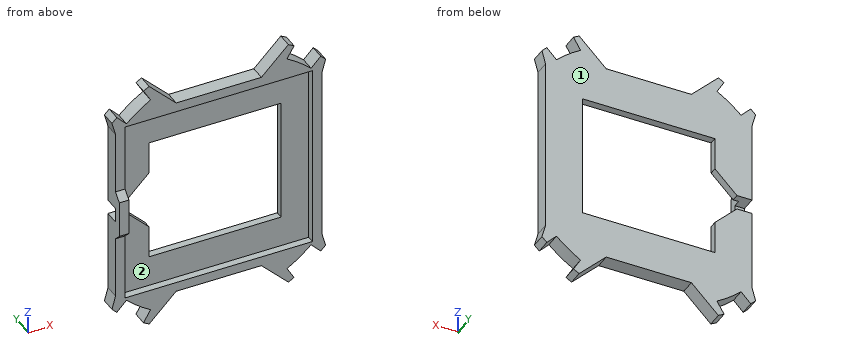
```python
from build123d import *

# Parameters (mm, degrees)
BOSS_EXTRUDE3_DEPTH      = 1
BOSS_EXTRUDE3_DEPTH_BACK = 1
SKETCH3_W                = 18
SKETCH3_H                = 17
CUT_EXTRUDE1_DEPTH       = 23.944525539
SKETCH3_4_W              = 25.5
SKETCH3_4_H              = 25.5
SKETCH3_4_W_2            = 18
SKETCH3_4_H_2            = 17
CUT_EXTRUDE3_DEPTH       = 23.944525539
CUT_EXTRUDE4_DEPTH       = 23.944525539
CUT_EXTRUDE4_DEPTH_BACK  = 23.944525539
SKETCH4_W                = 16
SKETCH4_H                = 2
CHAMFER1_SIZE            = 3
SKETCH6_W                = 5
SKETCH6_H                = 1
BOSS_EXTRUDE5_DEPTH      = 1.3
CHAMFER2_SIZE            = 1


with BuildPart() as part:
    # Sketch2 → Boss-Extrude3 (new, two sides: drawn at the far end of the back side and taken through both)
    with BuildSketch(Plane(origin=(0, -16.832566415, 0), x_dir=(1, 0, 0), z_dir=(0, 1, 0)).offset(-BOSS_EXTRUDE3_DEPTH_BACK)):
        with BuildLine():
            Line((14.05, -12.05), (14.05, 12.05))
            Line((14.05, 12.05), (14.538378439, 13.872653149))
            ThreePointArc((14.538378439, 13.872653149), (14.210517369, 14.208312678), (13.874908715, 14.536225824))
            Line((13.874908715, 14.536225824), (12.56303347, 13.16182292))
            ThreePointArc((12.56303347, 13.16182292), (10.992315824, 14.499392587), (9.280277793, 15.650553876))
            Line((9.280277793, 15.650553876), (10.249356378, 17.284838642))
            ThreePointArc((10.249356378, 17.284838642), (9.863353095, 17.507975862), (9.47249431, 17.72249431))
            Line((9.47249431, 17.72249431), (5.8, 14.05))
            Line((5.8, 14.05), (-5.8, 14.05))
            Line((-5.8, 14.05), (-9.47249431, 17.72249431))
            ThreePointArc((-9.47249431, 17.72249431), (-9.863353095, 17.507975862), (-10.249356378, 17.284838642))
            Line((-10.249356378, 17.284838642), (-9.280277793, 15.650553876))
            ThreePointArc((-9.280277793, 15.650553876), (-10.992315824, 14.499392587), (-12.56303347, 13.16182292))
            Line((-12.56303347, 13.16182292), (-13.874908715, 14.536225824))
            ThreePointArc((-13.874908715, 14.536225824), (-14.210517369, 14.208312678), (-14.538378439, 13.872653149))
            Line((-14.538378439, 13.872653149), (-14.05, 12.05))
            Line((-14.05, 12.05), (-14.05, -12.05))
            Line((-14.05, -12.05), (-14.538378439, -13.872653149))
            ThreePointArc((-14.538378439, -13.872653149), (-14.210517369, -14.208312678), (-13.874908715, -14.536225824))
            Line((-13.874908715, -14.536225824), (-12.56303347, -13.16182292))
            ThreePointArc((-12.56303347, -13.16182292), (-10.992315824, -14.499392587), (-9.280277793, -15.650553876))
            Line((-9.280277793, -15.650553876), (-10.249356378, -17.284838642))
            ThreePointArc((-10.249356378, -17.284838642), (-9.863353095, -17.507975862), (-9.47249431, -17.72249431))
            Line((-9.47249431, -17.72249431), (-5.8, -14.05))
            Line((-5.8, -14.05), (5.8, -14.05))
            Line((5.8, -14.05), (9.47249431, -17.72249431))
            ThreePointArc((9.47249431, -17.72249431), (9.863353095, -17.507975862), (10.249356378, -17.284838642))
            Line((10.249356378, -17.284838642), (9.280277793, -15.650553876))
            ThreePointArc((9.280277793, -15.650553876), (10.992315824, -14.499392587), (12.56303347, -13.16182292))
            Line((12.56303347, -13.16182292), (13.874908715, -14.536225824))
            ThreePointArc((13.874908715, -14.536225824), (14.210517369, -14.208312678), (14.538378439, -13.872653149))
            Line((14.538378439, -13.872653149), (14.05, -12.05))
        make_face()
    extrude(amount=BOSS_EXTRUDE3_DEPTH + BOSS_EXTRUDE3_DEPTH_BACK)

    # Sketch3 → Cut-Extrude1 (cut, through all)
    with BuildSketch(Plane(origin=(0, -16.832566415, 0), x_dir=(1, 0, 0), z_dir=(0, 1, 0))):
        Rectangle(SKETCH3_W, SKETCH3_H)
    extrude(amount=CUT_EXTRUDE1_DEPTH, mode=Mode.SUBTRACT)

    # Sketch3<4> → Cut-Extrude3 (cut, through all)
    # profile 1 of 2: a face of its own
    with BuildSketch(Plane(origin=(0, -16.832566415, 0), x_dir=(1, 0, 0), z_dir=(0, 1, 0))):
        Rectangle(SKETCH3_4_W, SKETCH3_4_H)
        Rectangle(SKETCH3_4_W_2, SKETCH3_4_H_2, mode=Mode.SUBTRACT)
    # profile 2 of 2: a face of its own
    with BuildSketch(Plane(origin=(0, -16.832566415, 0), x_dir=(1, 0, 0), z_dir=(0, 1, 0))):
        Rectangle(SKETCH3_4_W_2, SKETCH3_4_H_2)
    extrude(amount=-CUT_EXTRUDE3_DEPTH, mode=Mode.SUBTRACT)

    # Sketch4 → Cut-Extrude4 (cut, two sides: drawn at the far end of the back side and taken through both)
    with BuildSketch(Plane(origin=(0, -16.832566415, 0), x_dir=(1, 0, 0), z_dir=(0, 1, 0)).offset(-CUT_EXTRUDE4_DEPTH_BACK)):
        with Locations((-13.844488576, 0)):
            Rectangle(SKETCH4_W, SKETCH4_H)
    extrude(amount=CUT_EXTRUDE4_DEPTH + CUT_EXTRUDE4_DEPTH_BACK, mode=Mode.SUBTRACT)

    # Chamfer1
    chamfer1_edges = [part.edges().sort_by_distance(p)[0] for p in [
        (-9, -16.332566415, -1),
        (-9, -16.332566415, 1),
    ]]
    chamfer(chamfer1_edges, length=CHAMFER1_SIZE)

    # Sketch6 → Boss-Extrude5 (add)
    with BuildSketch(Plane.ZY.offset(14.05)):
        with Locations((0, -18.332566415)):
            Rectangle(SKETCH6_W, SKETCH6_H)
    extrude(amount=-BOSS_EXTRUDE5_DEPTH)

    # Chamfer2
    chamfer2_edges = [part.edges().sort_by_distance(p)[0] for p in [
        (-13.4, -17.832566415, 2.5),
        (-13.4, -17.832566415, -2.5),
    ]]
    chamfer(chamfer2_edges, length=CHAMFER2_SIZE - 0.0001)  # a hair under: the kernel refuses the full size


solid = part.part
```
Here's how the part is built. I have some questions about the finished solid (model axes, mm). Face numbers are marked on the shaded views. Coordinates: 2 decimals unless noted, no trailing zeros. Order: outer loops, then holes, each group sorted by start corner. A loop starts at its lowest first (then second) coordinate and runs counter-clockwise, first axis right, second up.
Item 1: If we section it at C-C, the plane z = -11: List the corners of the cut face in (x, y) for me, then the cut area to 3 significant figures.
Response values:
outline: (-14.05, -17.83) - (-12.75, -17.83) - (-12.75, -16.83) - (12.75, -16.83) - (12.75, -17.83) - (14.05, -17.83) - (14.05, -15.83) - (-14.05, -15.83) - close
area: 30.7 mm2
Item 2: I need wall thicknesses on probe 1 along X at (y, z) = (-17.2, 5); probe 2 along Y at (x, z) = (-10, 10.5). Which ranges of each line are inside material? Lowest first, please.
Response values:
probe 1: x = -14.05 to -12.75, 12.75 to 14.05
probe 2: y = -16.83 to -15.83
Item 3: I'm going to push flat-ended pins straight in: pin 1 Ø0.8 at (x, y) = (5.5, -17) entering from -Z; pin 2 Ø1.1 at (y, z) = (-17.5, -2.5) entering from -X; pin 3 Ø14.5 at (x, z) = (1, 6) entering from -Y; pin 4 Ø3 at (x, z) = (-6.5, -3.5) entering from +Y. Where does each tip first touch, or does it pass through?
Response values:
pin 1: stops at z = -14.15
pin 2: stops at x = -14.05
pin 3: stops at y = -17.83
pin 4: passes through
Item 4: If we section it at A-A, the plane z = 5.5: List the corners of the cut face in (x, y) for me.
Response values:
outline: (-14.05, -17.83) - (-12.75, -17.83) - (-12.75, -16.83) - (-9, -16.83) - (-9, -15.83) - (-14.05, -15.83) - close; (9, -16.83) - (12.75, -16.83) - (12.75, -17.83) - (14.05, -17.83) - (14.05, -15.83) - (9, -15.83) - close
Item 5: If we section it at B-B, the plane x = -1.75: List the corners of the cut face in (y, z) for me, then the cut area to 3 significant figures.
Response values:
outline: (-17.83, -14.05) - (-15.83, -14.05) - (-15.83, -8.5) - (-16.83, -8.5) - (-16.83, -12.75) - (-17.83, -12.75) - close; (-17.83, 12.75) - (-16.83, 12.75) - (-16.83, 8.5) - (-15.83, 8.5) - (-15.83, 14.05) - (-17.83, 14.05) - close
area: 13.7 mm2
Item 6: If we section it at D-D, the plane x = 10.75: List the corners of the cut face in (y, z) for me.
Response values:
outline: (-17.83, -14.68) - (-15.83, -14.68) - (-15.83, 14.68) - (-17.83, 14.68) - (-17.83, 12.75) - (-16.83, 12.75) - (-16.83, -12.75) - (-17.83, -12.75) - close
Item 7: Thinking about a two-plate mould opening in X: for the marked faces 1 and 2, which applies, pulls with the +X half, pulls with the -X half, needs draft (parallel to the pull), parting line crosses it, or undercut?
Response values:
face 1: needs draft
face 2: undercut
